Here's how the part is built. I have some questions about the finished solid (model axes, mm). A direction names the side the tool comes from. Round coordinates to 2 decimals unless told otherwise and drop trailing zeros. Loops run counter-clockwise (first coordinate to the right, second up) from the corner with the lowest first, then second, coordinate; pieces in that order, holes last. Notation, with made-up numbers: M 70.5,78.5 L 86.5,78.5 A20 ccw 86.5,86.5 Z; hole C 68,71 d2. An arc over 180 degrees is marked long. Answer as a JSON object with one key per item and string values.
Autodesk Inventor part; units mm, degrees
ref_plane "Work Plane1" through (104.775, 0, 0) normal (0, 0, -1) x (1, 0, 0)
ref_plane "YZ Plane" through (0, 0, 0) normal (1, 0, 0) x (0, 1, 0)
ref_plane "XZ Plane" through (0, 0, 0) normal (0, 1, 0) x (-1, 0, 0)
sketch "Sketch1" plane through (0, 0, 0) normal (0, 0, 1) x (1, 0, 0)
  line L0 (12.7, 0) -> (12.7, 1.7526)
  line L1 (12.7, 1.7526) -> (4.4483, 1.7526)
  line L2 (4.4483, 1.7526) -> (2.4638, 1.7526)
  line L3 (0, 3.3401) -> (0, 1.1438)
  line L4 (0, 1.1438) -> (1.6764, 1.1438)
  line L5 (1.6764, 1.1438) -> (2.3368, 0)
  line L6 (2.3368, 0) -> (12.7, 0)
  line L7 (0, 3.3401) -> (0.6376, 3.3401)
  line L8 (0.6376, 3.3401) -> (2.4638, 1.7526)
  line L9 (2.4638, 1.7526) -> (2.4638, 1.7526)
  line L10 (4.4483, 1.7526) -> (2.4638, 1.7526) construction
  line L11 (2.4638, 1.7526) -> (2.4638, 1.7526)
  line L12 (-2.54, 0) -> (15.24, 0)
  line L13 (0, -0.668) -> (0, 4.0081)
  dimension "d0" = 12.7
  dimension "d1" = 8.2517
  dimension "d2" = 1.6764
  dimension "d3" = 3.5052
  dimension "d6" = 2.4638
  dimension "d7" = 41
  dimension "d8" = 2.2877
  dimension "d9" = 60
  dimension "d10" = 6.6802
  dimension "d11" = 3.5052
  dimension "d12" = 1.9845
revolve "Body" add sketch "Sketch1" angle 360 about axis through (2.3368, 0, 0) along (1, 0, 0) contours L6 L5 L4 L3 L7 L8 L2 L1 L0
sketch "Sketch2" plane through (0, 0, 0) normal (-1, 0, 0) x (0, 0, 1)
  circle A0 centre (0, 0) radius 1.1438
  line L0 (0, -4.6761) -> (0, 4.6761)
  line L1 (-4.6761, 0) -> (4.6761, 0)
  line L2 (1.1438, 0) -> (0.5719, -0.9906)
  line L3 (0.5719, -0.9906) -> (-0.5719, -0.9906)
  line L4 (-0.5719, -0.9906) -> (-1.1438, 0)
  line L5 (-1.1438, 0) -> (-0.5719, 0.9906)
  line L6 (-0.5719, 0.9906) -> (0.5719, 0.9906)
  line L7 (0.5719, 0.9906) -> (1.1438, 0)
  point P0 (0, 1.1438)
extrude "Slot" add sketch "Sketch2" against normal up to next contours L7 A0 | A0 L2 | L6 L0 A0 | A0 L0 L3 | L0 L6 A0 | A0 L3 L0 | L4 A0 | A0 L5
thread "Thread"
chamfer "Chamfer1" distance 0.4724 distance2 0.9449 1 edges at (12.7, -1.7526, 0) measured on face at (12.7, 0.5842, 0.7748)
ref_plane "Work Plane1" through (104.775, 0, 0) normal (0, 0, -1) x (1, 0, 0)
equation "\"d15\" = GEL"
equation "\"d17\" = -0.5 * SPD + 0.5 * GD"
equation "\"d18\" = GUL"
equation "\"d0\" = NLG"
equation "\"d1\" = GEL"
equation "\"d2\" = INTI"
equation "\"d3\" = GD"
equation "\"d6\" = KOH"
equation "\"d7\" = 0.5 * SEWI"
equation "\"d8\" = 1.1547 * SW"
equation "\"d10\" = KOD"
equation "\"d11\" = BDM"
equation "\"d12\" = GAL"
equation "\"NLG\" = 12.7"
equation "\"INTI\" = 1.6764"
equation "\"GEL\" = 8.2517"
equation "\"GAL\" = 1.9845"
equation "\"KOH\" = 2.4638"
equation "\"KOD\" = 6.6802"
equation "\"GUL\" = 0.94488"
equation "\"SPD\" = 2.56032"
equation "\"BDM\" = NND"
equation "\"GD\" = NND"
equation "\"SEWI\" = 82deg"
equation "\"SW\" = 1.9812"
equation "\"TOA\" = 30deg"
equation "\"GD1\" = SPD"
equation "\"THREADDIA\" = 3.5052"
equation "\"HHPTC\" = 0.79375"
equation "\"NND\" = 3.5052"
equation "\"E0\" = 1.155 * SW"
properties part number "ANSI B18.3 - 6-32 UNC x 0.5, HSFCHCSI" material "Steel, Mild"
Item 1: If we mould it in two halves opening along Y, with no side actions, what happens to faces 4 (the face through (0.87, -0.49, 0.86)), 5 (the face through (2.35, -0.4, 1.81)), 6 (the face through (12.7, 0, 0))? For each: pulls with the +Y half, pulls with the -Y half, needs draft (parallel to the pull), parting line crosses it, or undercut.
Resolved:
{"face 4": "undercut", "face 5": "parting line crosses it", "face 6": "needs draft"}
Item 2: On a 3-axis mill with a long thin cutter (end or side, diameter ignored), from which of +Z, -Z, +X, -X, +Y, -Y can I reach the whole of each face in a straight line? I mean faces 1 (the face through (0, -1, -1)), 2 (the face through (7.04, 1.67, -0.53)), 3 (the face through (0.87, 0.49, -0.86)). Say none if no direction works.
Resolved:
{"face 1": "+Z, -Z, -X, +Y, -Y", "face 2": "+X", "face 3": "-X"}
Item 3: I'm going to push flat-ended pins straight in: pin 1 Ø1 at (x, z) = (5.5, 0.5) entering from -Y; pin 2 Ø1 at (x, y) = (11, 0.5) entering from +Z; pin 3 Ø1.5 at (x, z) = (5, 1) entering from -Y. Where does each tip first touch, or does it pass through?
Resolved:
{"pin 1": "y = -1.75", "pin 2": "z = 1.75", "pin 3": "y = -1.73"}
Item 4: Please list where these lines run through material, in increasing order: probe 1 along X at (y, z) = (0, -3); probe 2 along Y at (x, z) = (8, 0.5); probe 3 along X at (y, z) = (-0.25, -0.75). Write a range as from..to.
Resolved:
{"probe 1": "0..1.03", "probe 2": "-1.68..1.68", "probe 3": "1.88..12.7"}
Item 5: I want a section at A-A, the plane x = 1. Please give me the cut outline in (y, z), then the cut area to 3 significant figures.
Resolved:
{"outline": "C 0,0 d6.05; hole M -0.99,-0.57 L 0,-1.14 L 0.99,-0.57 L 0.99,0.57 L 0,1.14 L -0.99,0.57 Z", "area": "25.3 mm²"}
Item 6: I want a section at B-B, the plane x = 4. Please give me the cut outline in (y, z), then the cut area to 3 significant figures.
Resolved:
{"outline": "C 0,0 d3.51", "area": "9.65 mm²"}
